from build123d import *

# Parameters (mm, degrees)
F1_DEPTH             = 34.2
F2_W                 = 34.2
F2_H                 = 34.2
F3_DEPTH             = 34.2
F4_W                 = 28.2
F4_H                 = 28.2
F5_DEPTH             = 31.2
F8_D                 = 3.3
F8_DEPTH             = 25
F8_CSINK_D           = 6.72
F8_CSINK_ANGLE       = 90
F8_TIP               = 0.9914200214
F8_ON_F7_D           = 3.3
F8_ON_F7_DEPTH       = 25
F8_ON_F7_CSINK_D     = 6.72
F8_ON_F7_CSINK_ANGLE = 90
F8_ON_F7_TIP         = 0.9914200214
F10_D                = 5.5
F10_DEPTH            = 25
F10_TIP              = 1.6523667023
F11_R                = 5
F12_W                = 28.2
F12_H                = 28.2
F13_DEPTH            = 31.2
F14_R                = 1.49999


# Not quite as in the source:
# - a fillet or chamfer is up to 0.001 mm smaller than in the source, because OpenCascade refuses the exact size


with BuildPart() as f1:
    # F0 (on Top) → F1 (new body)
    with BuildSketch(Plane.XY):
        with BuildLine():
            Line((0, 0), (-8, 0))
            Line((-8, 0), (-8, -4))
            ThreePointArc((-8, -4), (-4, -8), (0, -4))
            Line((0, -4), (0, 0))
        make_face()
        Polygon((-34.2, 0), (-8, 0), (0, 0), (0, 34.2), (-34.2, 34.2), align=None)
    extrude(amount=F1_DEPTH)

    # F2 (on face) → F3 (join)
    with BuildSketch(Plane(origin=(-34.2, 0, 0), x_dir=(0, -1, 0), z_dir=(-1, 0, 0))):
        with Locations((-17.1, 17.1)):
            Rectangle(F2_W, F2_H)
    extrude(amount=F3_DEPTH)

    # F4 (on face) → F5 (cut)
    with BuildSketch(Plane(origin=(-68.4, 0, 0), x_dir=(0, -1, 0), z_dir=(-1, 0, 0))):
        with Locations((-17.1, 17.1)):
            Rectangle(F4_W, F4_H)
    extrude(amount=-F5_DEPTH, mode=Mode.SUBTRACT)

    # F8
    with Locations(Plane(origin=(0, 34.2, 0), x_dir=(-1, 0, 0), z_dir=(0, 1, 0))):
        with Locations((17.05, 17.1), (51.35, 17.1)):
            CounterSinkHole(F8_D / 2, F8_CSINK_D / 2, depth=F8_DEPTH, counter_sink_angle=F8_CSINK_ANGLE)
            with Locations((0, 0, -(F8_DEPTH + F8_TIP / 2))):  # 118° drill point
                Cone(0, F8_D / 2, F8_TIP, mode=Mode.SUBTRACT)

    # F8 on F7
    with Locations(Plane(origin=(-37.2, 0, 0), x_dir=(0, -1, 0), z_dir=(-1, 0, 0))):
        with Locations((-17.1, 17.1)):
            CounterSinkHole(F8_ON_F7_D / 2, F8_ON_F7_CSINK_D / 2, depth=F8_ON_F7_DEPTH, counter_sink_angle=F8_ON_F7_CSINK_ANGLE)
            with Locations((0, 0, -(F8_ON_F7_DEPTH + F8_ON_F7_TIP / 2))):  # 118° drill point
                Cone(0, F8_ON_F7_D / 2, F8_ON_F7_TIP, mode=Mode.SUBTRACT)

    # F10
    with Locations(Plane.XY.offset(34.2)):
        with Locations((-4, -4)):
            Hole(F10_D / 2, depth=F10_DEPTH)
            with Locations((0, 0, -(F10_DEPTH + F10_TIP / 2))):  # 118° drill point
                Cone(0, F10_D / 2, F10_TIP, mode=Mode.SUBTRACT)

    # F11
    f11_edges = [f1.edges().sort_by_distance(p)[0] for p in [
        (-8, 0, 17.1),
    ]]
    fillet(f11_edges, radius=F11_R)

    # F12 (on face) → F13 (cut)
    with BuildSketch(Plane(origin=(0, 0, 0), x_dir=(1, 0, 0), z_dir=(0, 0, -1))):
        with Locations((-17.1, -17.1)):
            Rectangle(F12_W, F12_H)
    extrude(amount=-F13_DEPTH, mode=Mode.SUBTRACT)

    # F14 (radius 1.5 in the source; OpenCascade refuses exactly that, so slightly less here)
    f14_edges = [f1.edges().sort_by_distance(p)[0] for p in [
        (-31.2, 17.1, 0),
        (-17.1, 3, 0),
        (-3, 17.1, 0),
        (-17.1, 31.2, 0),
        (-34.2, 34.2, 0),
        (-40.672136, 0, 0),
        (0, 15.1, 0),
        (-68.4, 17.1, 0),
        (-68.4, 0, 17.1),
        (-68.4, 17.1, 34.2),
        (-68.4, 34.2, 17.1),
        (-68.4, 17.1, 31.2),
        (-68.4, 3, 17.1),
        (-68.4, 17.1, 3),
        (-68.4, 31.2, 17.1),
        (-40.672136, 0, 34.2),
        (-34.2, 34.2, 34.2),
        (0, 15.1, 34.2),
        (0, 34.2, 17.1),
    ]]
    fillet(f14_edges, radius=F14_R)


solid = f1.part
The model under review builds one solid part; all positions refer to its coordinate system, in mm. A direction names the side the tool comes from. Coordinates: 2 decimals unless noted, no trailing zeros. Write each loop counter-clockwise with the first axis right and the second up, starting at its lowest first coordinate (ties: lowest second). Pieces come first, ordered by that corner, then holes. Notation, with made-up numbers: M 35.25,11.25 L 45.25,11.25 A17 ccw 45.25,37.25 Z; hole C -39.75,78 d10. An arc over 180 degrees is marked long. Put each result on its own line as item: value.
1) For faces 4 (the cylindrical face through (-39.54, 0.45, 33.77)), 5 (the flat face through (-20, 31.2, 16)), 6 (the cylindrical face through (-17.41, 31.84, 15.49)), 7 (the cylindrical face through (-3.404, -6.685, 21.525)), list the 3-axis set-ups (+Z, -Z, +X, -X, +Y, -Y) from which the entire face can be reached by the end or side of a thin tool; tool diameter is ignored.
Computed:
face 4: +Z, -X, -Y
face 5: -Z
face 6: +Y
face 7: +Z
2) Wall thickness on probe 1 along Y at (x, z) = (-4, 25); probe 2 along X at (y, z) = (30.5, 29.5); probe 3 along Y at (x, z) = (-45, 19): over which ranges is each line inside the solid? List them lowest first. Write a range as [from, to].
Computed:
probe 1: y = [-8, -6.75], [-1.25, 3], [31.2, 34.2]
probe 2: x = [-37.2, -31.2], [-3, 0]
probe 3: y = [0, 3], [31.2, 34.2]
3) Clearance check with flat-ended pins moving along their axes: pin 1 Ø14 at (x, z) = (-17.5, 21) entering from -Y; pin 2 Ø3.5 at (x, y) = (-4, -4) entering from +Z; pin 3 Ø10 at (x, z) = (-55.5, 4.5) entering from -Y. State where each tip first meets the part, or that it passes through.
Computed:
pin 1: stops at y = -0.64
pin 2: stops at z = 8.6
pin 3: stops at y = 0
4) Draft analysis for pull direction Z (two halves, no side actions). For faces 1 (the cylindrical face through (-16.88, 31.65, 0.43)), 2 (the cylindrical face through (-4, -8, 17)), 3 (the cylindrical face through (-67.97, 2.55, 17.32)), state which applies: released by +Z, released by -Z, zero draft, split by the parting line, or undercut.
Computed:
face 1: released by -Z
face 2: zero draft
face 3: undercut
5) Add section D-D on x = -41.5. Give the boundary of the cut face in (y, z).
Computed:
outline: M 0,1.5 A1.5 ccw 1.5,0 L 32.7,0 A1.5 ccw 34.2,1.5 L 34.2,32.7 A1.5 ccw 32.7,34.2 L 1.5,34.2 A1.5 ccw 0,32.7 Z; hole M 3,3 L 31.2,3 L 31.2,31.2 L 3,31.2 Z
6) Add section C-C on z = 17.1. State how many separate pieces and enclosed holes the cut face has, then the cut area to 3 significant figures.
Computed:
separate pieces: 3
enclosed holes: 1
area: 652 mm2
